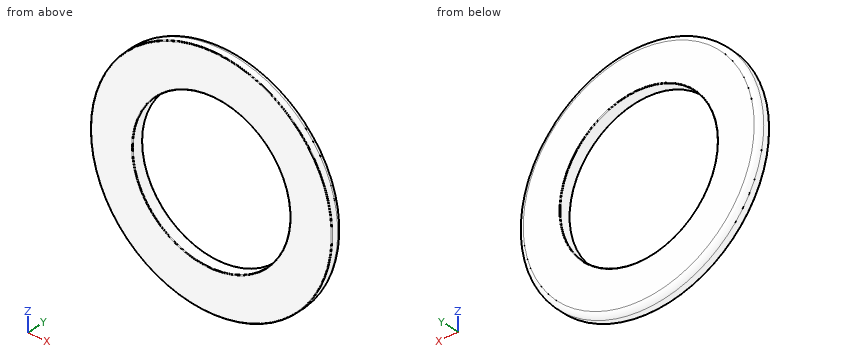
Autodesk Inventor part; units mm, degrees
ref_plane "YZ Plane" through (0, 0, 0) normal (1, 0, 0) x (0, 1, 0)
ref_plane "XZ Plane" through (0, 0, 0) normal (0, 1, 0) x (-1, 0, 0)
ref_plane "XY Plane" through (0, 0, 0) normal (0, 0, 1) x (1, 0, 0)
sketch "Skizze1" plane through (0, 0, 0) normal (0, 1, 0) x (-1, 0, 0)
  circle A0 centre (0, 0) radius 225.5
  circle A1 centre (0, 0) radius 345.5
  dimension "d0" = 120
  dimension "d1" = 451
extrude "Extrusion1" add sketch "Skizze1" along normal blind 35
fillet "Rundung1" radius 15 1 edges at (345.5, 35, 0)
fillet "Rundung2" radius 2 1 edges at (225.5, 35, 0)
fillet "Rundung3" radius 2 2 edges at (345.5, 0, 0) (225.5, 0, 0)
properties part number "Surround"
Verification items for the finished model (mm, model axes). Give positions to 0.01 mm unless a question says otherwise; leave off trailing zeros. Loops run counter-clockwise (first coordinate to the right, second up) from the corner with the lowest first, then second, coordinate; pieces in that order, holes last.
1. Section check B-B, the plane x = 0. Enter the section's corners in (y, z), then the cut area to 3 significant figures.
2. Section check A-A, the plane z = 0. Enter the section's corners in (x, y).
3. Thickness scan on line 1 (Z direction, x = 0, y = 22); line 2 (Z direction, x = 0, y = 12.5); line 3 (X direction, y = 11.5, z = 108.5). Record the ranges inside material, lowest first.
4. Go/stop test with flat-tipped pins: pin 1 Ø6 at (x, y) = (-63.5, 17) entering from -Z; pin 2 Ø4 at (x, y) = (-160, 6) entering from -Z; pin 3 Ø6 at (x, y) = (99, 17) entering from -Z. Record where each tip stops, or that it passes through.
5. Section check C-C, the plane y = 14. Enter the section's corners in (x, z), then the cut area to 3 significant figures.
Geometry says:
1. outline: (0, -343.5) arc R2 ccw to (2, -345.5) - (20, -345.5) arc R15 ccw to (35, -330.5) - (35, -227.5) arc R2 ccw to (33, -225.5) - (2, -225.5) arc R2 ccw to (0, -227.5) - close; (0, 227.5) arc R2 ccw to (2, 225.5) - (33, 225.5) arc R2 ccw to (35, 227.5) - (35, 330.5) arc R15 ccw to (20, 345.5) - (2, 345.5) arc R2 ccw to (0, 343.5) - close
1. area: 8,300 mm2
2. outline: (-345.5, 2) arc R2 ccw to (-343.5, 0) - (-227.5, 0) arc R2 ccw to (-225.5, 2) - (-225.5, 33) arc R2 ccw to (-227.5, 35) - (-330.5, 35) arc R15 ccw to (-345.5, 20) - close; (225.5, 2) arc R2 ccw to (227.5, 0) - (343.5, 0) arc R2 ccw to (345.5, 2) - (345.5, 20) arc R15 ccw to (330.5, 35) - (227.5, 35) arc R2 ccw to (225.5, 33) - close
3. line 1: z = -345.37 to -225.5, 225.5 to 345.37
3. line 2: z = -345.5 to -225.5, 225.5 to 345.5
3. line 3: x = -328.02 to -197.68, 197.68 to 328.02
4. pin 1: stops at z = -340.16
4. pin 2: stops at z = -307.26
4. pin 3: stops at z = -331.89
5. outline: circle Ø691 at (0, 0); hole circle Ø451 at (0, 0)
5. area: 215,000 mm2
